from build123d import *

# Parameters (mm, degrees)
F1_DEPTH = 6.35
F2_R     = 1.6002


with BuildPart() as f1:
    # F0 (on Top) → F1 (new body)
    with BuildSketch(Plane.XY):
        Polygon((-60.581866, 0), (0, 0), (15.618134, 0), (15.618134, 15.24), (-22.481866, 15.24), (-22.481866, 27.432), (-60.581866, 6.858), align=None)
    extrude(amount=F1_DEPTH)

    # F2
    f2_edges = [f1.edges().sort_by_distance(p)[0] for p in [
        (-60.581866, 6.858, 3.175),
        (-60.581866, 0, 3.175),
        (-22.481866, 27.432, 3.175),
        (15.618134, 15.24, 3.175),
        (15.618134, 0, 3.175),
    ]]
    fillet(f2_edges, radius=F2_R)


solid = f1.part
CAD build for the part. Positions are in the model's coordinates, mm. A direction names the side the tool comes from. Round coordinates to 2 decimals unless told otherwise and drop trailing zeros. Loops run counter-clockwise (first coordinate to the right, second up) from the corner with the lowest first, then second, coordinate; pieces in that order, holes last. Notation, with made-up numbers: (61, 75.25) - (112, 75.25) arc R12 ccw to (112, 85.25) - close; hole circle Ø4 at (48.25, 67.5). An arc over 180 degrees is marked (long way). Put each result on its own line as item: value.
1. 3-axis set-ups, long thin cutter, end or side, ignore diameter. For faces 1 (the flat face through (-22.482, 20, 3)), 2 (the cylindrical face through (-23.24, 26.11, 3.22)): which of +Z, -Z, +X, -X, +Y, -Y reach the whole face in a straight line?
Geometry check:
face 1: +Z, -Z, +X, +Y
face 2: +Z, -Z, +Y
2. Slice it at A-A on z = 4.75. List the corners of the cut face in (x, y), and give its area (3 significant figures).
Geometry check:
outline: (-60.58, 1.6) arc R1.6 ccw to (-58.98, 0) - (14.02, 0) arc R1.6 ccw to (15.62, 1.6) - (15.62, 13.64) arc R1.6 ccw to (14.02, 15.24) - (-22.48, 15.24) - (-22.48, 24.75) arc R1.6 ccw to (-24.84, 26.16) - (-59.74, 7.31) arc R1.6 ccw to (-60.58, 5.9) - close
area: 1,230 mm²
3. Slice it at C-C on y = 21.75. List the corners of the cut face in (x, z).
Geometry check:
outline: (-33, 0) - (-22.48, 0) - (-22.48, 6.35) - (-33, 6.35) - close
4. Slice it at B-B on x = -18.5. List the corners of the cut face in (y, z), and give its area (3 significant figures).
Geometry check:
outline: (0, 0) - (15.24, 0) - (15.24, 6.35) - (0, 6.35) - close
area: 96.8 mm²
5. Pin check, flat tips, straight feed: P1, Ø3, axis at y = 21, z = 1, coming from the -X side; P2, Ø3, axis at x = -3.5, z = 3, coming from the +Y side. Stop position of each tip, or through.
Geometry check:
P1: x = -37.17
P2: y = 15.24
6. Wall check: line 1 (Y direction, x = -15.5, z = 2); line 2 (X direction, y = 9.5, z = 5); line 3 (X direction, y = 23.25, z = 5). Give the ranges that are in metal, low to high.
Geometry check:
line 1: 0 to 15.24
line 2: -55.69 to 15.62
line 3: -30.23 to -22.48
